Here's how the part is built. I have some questions about the finished solid (model axes, mm). Round coordinates to 2 decimals unless told otherwise and drop trailing zeros. Order: outer loops, then holes, each group sorted by start corner. A loop starts at its lowest first (then second) coordinate and runs counter-clockwise, first axis right, second up. Notation, with made-up numbers: (15, 68) -> (61, 68) arc R26 cw to (61, 98) -> close; hole circle Ø9 at (3.5, 87). An arc over 180 degrees is marked (long way). Use a Markdown table: item, result. Add a question column.
(1) I want a section at A-A, the plane z = -0.95. Give the number of separate pieces and of enclosed holes in the cut face, then the cut area to 3 significant figures.
(2) If I drill on probe 1 along X at (y, z) = (503.64, -0.9); probe 2 along Y at (x, z) = (42.5, -0.5); probe 3 along X at (y, z) = (184.1, -1.2), over which ranges is the centre line in solid material (lowest first)?
(3) I want a section at C-C, the plane y = 60. Please give me the cut outline in (x, z).
(4) I want a section at B-B, the plane y = 216. Please give me the cut outline in (x, z), then the cut area to 3 significant figures.
from build123d import *

# Parameters (mm, degrees)
ESBO_O1_R          = 3.5
FLANGE_BASE1_DEPTH = 2


# Sheet-metal steps are written as plain solids
with BuildPart() as part:
    # Esboço1 → Flange-base1 (new body)
    with BuildSketch(Plane.XY):
        with BuildLine():
            Line((-44.875, 0), (44.875, 0))
            ThreePointArc((44.875, 0), (48.887773278, 1.539321731), (50.84156352, 5.367449793))
            Line((50.84156352, 5.367449793), (109, 553.95))
            Line((109, 553.95), (109, 616.76))
            ThreePointArc((109, 616.76), (107.242640687, 621.002640687), (103, 622.76))
            Line((103, 622.76), (-103, 622.76))
            ThreePointArc((-103, 622.76), (-107.242640687, 621.002640687), (-109, 616.76))
            Line((-109, 616.76), (-109, 553.95))
            Line((-109, 553.95), (-50.84156352, 5.367449793))
            ThreePointArc((-50.84156352, 5.367449793), (-48.887773278, 1.539321731), (-44.875, 0))
        make_face()
        with Locations((-98, 586.08)):
            Circle(ESBO_O1_R, mode=Mode.SUBTRACT)
        with Locations((98, 586.08)):
            Circle(ESBO_O1_R, mode=Mode.SUBTRACT)
        with Locations((-92.5, 503.64)):
            Circle(ESBO_O1_R, mode=Mode.SUBTRACT)
        with Locations((92.5, 503.64)):
            Circle(ESBO_O1_R, mode=Mode.SUBTRACT)
        with Locations((-75.56185023, 343.87)):
            Circle(ESBO_O1_R, mode=Mode.SUBTRACT)
        with Locations((-58.623700461, 184.1)):
            Circle(ESBO_O1_R, mode=Mode.SUBTRACT)
        with Locations((-41.685550691, 24.33)):
            Circle(ESBO_O1_R, mode=Mode.SUBTRACT)
        with Locations(Location((41.685550691, 24.33, 0), (0, 0, 180))):
            Circle(ESBO_O1_R, mode=Mode.SUBTRACT)
        with Locations(Location((58.623700461, 184.1, 0), (0, 0, 180))):
            Circle(ESBO_O1_R, mode=Mode.SUBTRACT)
        with Locations(Location((75.56185023, 343.87, 0), (0, 0, 180))):
            Circle(ESBO_O1_R, mode=Mode.SUBTRACT)
    extrude(amount=-FLANGE_BASE1_DEPTH)


solid = part.part
Taken from the geometry:
| question | item | result |
|---|---|---|
| 1 | separate pieces | 1 |
| 1 | enclosed holes | 10 |
| 1 | area | 103,000 mm2 |
| 2 | probe 1 | x = -103.67 to -96, -89 to 89, 96 to 103.67 |
| 2 | probe 2 | y = 0 to 20.93, 27.73 to 622.76 |
| 2 | probe 3 | x = -69.79 to -62.12, -55.12 to 55.12, 62.12 to 69.79 |
| 3 | outline | (-56.63, -2) -> (56.63, -2) -> (56.63, 0) -> (-56.63, 0) -> close |
| 4 | outline | (-73.17, -2) -> (73.17, -2) -> (73.17, 0) -> (-73.17, 0) -> close |
| 4 | area | 293 mm2 |
